Verification items for this drawing (mm, ordinates from the low corner). A direction names the side the tool comes from. Round coordinates to 2 decimals unless told otherwise and drop trailing zeros. Write each loop counter-clockwise with the first axis right and the second up, starting at its lowest first coordinate (ties: lowest second). Pieces come first, ordered by that corner, then holes.
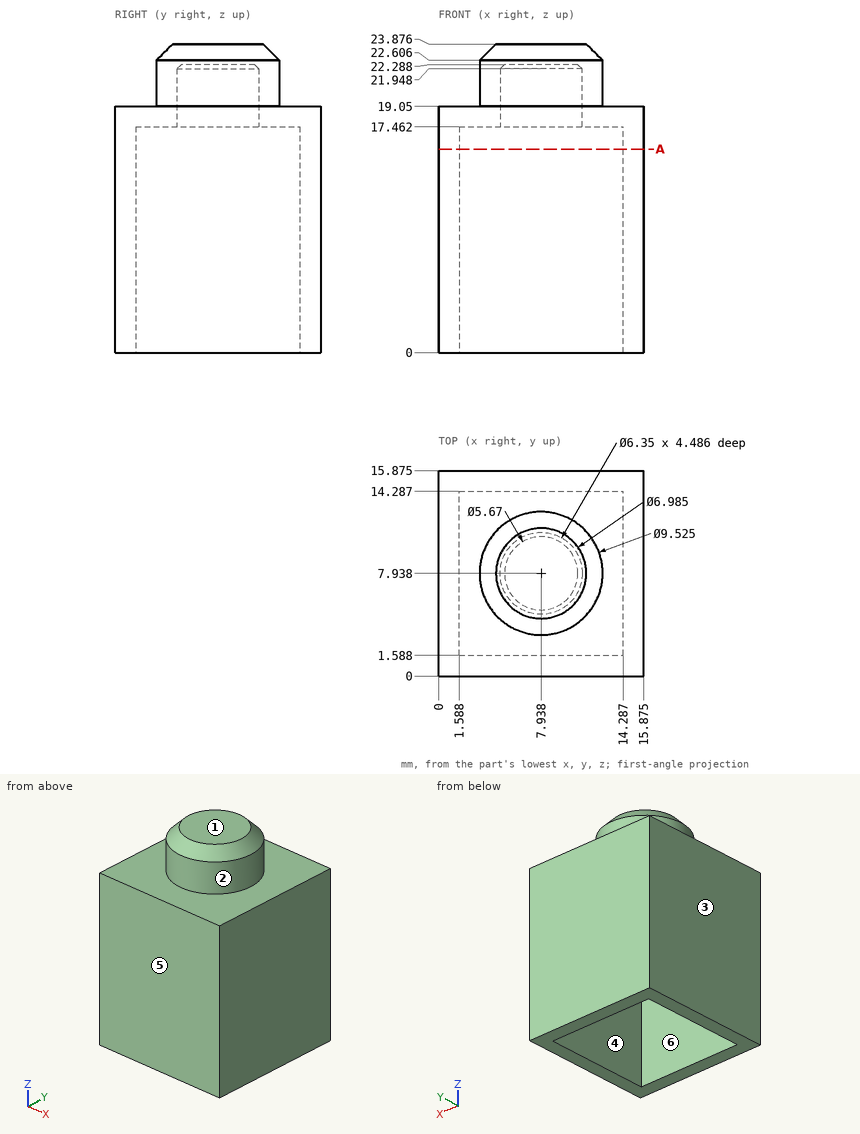
1. Scan lines: line 1 along Y through (x, z) = (3.75, 9.75) (1 decimal); line 2 along Z through (x, y) = (8, 1.75). Record each from-to range of solid material in increasing order.
2. Section check A-A (z = 15.75). Record the cut outline in (x, y) (1 decimal).
3. Release check for a two-part mould opening along Y. For the marked faces 3, 4, 5 and 6 record: +Y half, -Y half, draft (parallel to the pull), parting line (faces both ways), or undercut.
4. Depth check by flat-ended pin: pin 1 Ø2 at (x, y) = (12, 4.5) entering from +Z (1 decimal); pin 2 Ø4 at (x, y) = (10.5, 10) entering from -Z; pin 3 Ø4.5 at (x, y) = (8, 7.5) entering from -Z. Enter the tip coordinate at first touch or a pass-through.
5. Access from +Z, -Z, +X, -X, +Y, -Y to the whole of each face (thin tool, end or side, straight path). Record for the marked faces 1 and 2.
Results below:
1. line 1: y = 0 to 1.6, 14.3 to 15.9
1. line 2: z = 17.46 to 19.05
2. outline: (0, 0) - (15.9, 0) - (15.9, 15.9) - (0, 15.9) - close; hole (1.6, 1.6) - (14.3, 1.6) - (14.3, 14.3) - (1.6, 14.3) - close
3. face 3: draft
3. face 4: undercut
3. face 5: -Y half
3. face 6: undercut
4. pin 1: stops at z = 23
4. pin 2: stops at z = 17.46
4. pin 3: stops at z = 22.29
5. face 1: +Z, +X, -X, +Y, -Y
5. face 2: +Z
